```python
from build123d import *

# Parameters (mm, degrees)
F0_R     = 10
F1_DEPTH = 6
F2_DEPTH = 100
F3_R     = 2


with BuildPart() as f1:
    # F0 (on Front) → F1 (new body)
    with BuildSketch(Plane.XZ):
        Polygon((-80, 20), (-80, 0), (0, 0), (80, 0), (80, 20), (61.93496, 20), (17, 20), (-17, 20), (-61.93496, 20), align=None)
        with BuildLine():
            Line((-25.16937, 144.615068), (-80, 20))
            Line((-80, 20), (-61.93496, 20))
            ThreePointArc((-61.93496, 20), (-63.609916, 20.907058), (-63.76559, 22.805477))
            Line((-63.76559, 22.805477), (-18.83063, 124.930386))
            ThreePointArc((-18.83063, 124.930386), (-16.588454, 126.082109), (-15, 124.124909))
            Line((-15, 124.124909), (-15, 22))
            ThreePointArc((-15, 22), (-15.585786, 20.585786), (-17, 20))
            Line((-17, 20), (17, 20))
            ThreePointArc((17, 20), (15.585786, 20.585786), (15, 22))
            Line((15, 22), (15, 124.124909))
            ThreePointArc((15, 124.124909), (16.588454, 126.082109), (18.83063, 124.930386))
            Line((18.83063, 124.930386), (63.76559, 22.805477))
            ThreePointArc((63.76559, 22.805477), (63.609916, 20.907058), (61.93496, 20))
            Line((61.93496, 20), (80, 20))
            Line((80, 20), (25.16937, 144.615068))
            ThreePointArc((25.16937, 144.615068), (25.0428, 145.009), (25, 145.420546))
            Line((25, 145.420546), (25, 160))
            ThreePointArc((25, 160), (17.67767, 177.67767), (0, 185))
            ThreePointArc((0, 185), (-17.67767, 177.67767), (-25, 160))
            Line((-25, 160), (-25, 145.420546))
            ThreePointArc((-25, 145.420546), (-25.0428, 145.009), (-25.16937, 144.615068))
        make_face()
        with Locations((0, 160)):
            Circle(F0_R, mode=Mode.SUBTRACT)
    extrude(amount=F1_DEPTH)

    # F0 (on Front) → F2 (join)
    with BuildSketch(Plane.XZ):
        Polygon((-80, 20), (-80, 0), (0, 0), (80, 0), (80, 20), (61.93496, 20), (17, 20), (-17, 20), (-61.93496, 20), align=None)
    extrude(amount=F2_DEPTH)

    # F3
    f3_edges = [f1.edges().sort_by_distance(p)[0] for p in [
        (70.96748, -6, 20),
        (0, -6, 20),
        (-70.96748, -6, 20),
    ]]
    fillet(f3_edges, radius=F3_R)


solid = f1.part
```
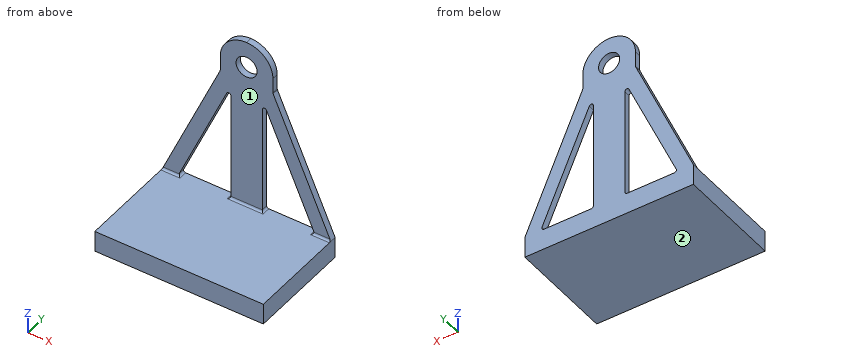
Geometry: final body of the model. Coordinates: model frame, mm. Face numbers are marked on the shaded views. A direction names the side the tool comes from. Round coordinates to 2 decimals unless told otherwise and drop trailing zeros. Write each loop counter-clockwise with the first axis right and the second up, starting at its lowest first coordinate (ties: lowest second). Pieces come first, ordered by that corner, then holes. Notation, with made-up numbers: M 38,-6.5 L 74,-6.5 A35 ccw 74,26.5 Z; hole C 36,89.25 d4. An arc over 180 degrees is marked long. Answer in a Markdown table with one row per item. Add a question column.
(1) Ray query, L1, parallel to Y at x = -14, z = 22.5; L2, parallel to Z at x = -46, y = -87.5; L3, parallel to Z at x = -11, y = -4.5. Return the intervals inside material, ascending.
(2) Reachability of the marked faces 1 and 2 from +Z, -Z, +X, -X, +Y, -Y: full face, straight path, thin tool, end or side. Return the list, or none.
(3) Contact query for flat-ended pins moving along their axis: pin 1 (6.5 mm diameter, centred on y = -1.5, z = 85.5, fed in from -X); pin 2 (6.5 mm diameter, centred on y = -3.5, z = 152.5, fed in from +X); pin 3 (5 mm diameter, centred on y = -2, z = 154, fed in from -X). Output: stop coordinate, or through.
(4) Cut plane C-C, the plane z = 135. Return the cut outline in (x, y).
(5) Cut plane A-A, the plane z = 106. Return the cut outline in (x, y).
(6) Cut plane D-D, the plane y = -31.5. Return the cut outline in (x, z).
(7) Cut plane B-B, the plane x = 31. Return the cut outline in (y, z).
Established:
| question | item | result |
|---|---|---|
| 1 | L1 | -6 to 0 |
| 1 | L2 | 0 to 20 |
| 1 | L3 | 0 to 182.45 |
| 2 | face 1 | +Z, +X, -X, -Y |
| 2 | face 2 | -Z, +X, -X, +Y, -Y |
| 3 | pin 1 | x = -52.61 |
| 3 | pin 2 | x = 25 |
| 3 | pin 3 | x = -25 |
| 4 | outline | M -29.4,-6 L 29.4,-6 L 29.4,0 L -29.4,0 Z |
| 5 | outline | M -42.16,-6 L -27.16,-6 L -27.16,0 L -42.16,0 Z; M -15,-6 L 15,-6 L 15,0 L -15,0 Z; M 27.16,-6 L 42.16,-6 L 42.16,0 L 27.16,0 Z |
| 6 | outline | M -80,0 L 80,0 L 80,20 L -80,20 Z |
| 7 | outline | M -100,0 L 0,0 L 0,20 L -100,20 Z; M -6,97.27 L 0,97.27 L 0,131.36 L -6,131.36 Z |
